Part model, mm, in its own coordinate system. Face numbers are marked on the shaded views. Round coordinates to 2 decimals unless told otherwise and drop trailing zeros. Loops run counter-clockwise (first coordinate to the right, second up) from the corner with the lowest first, then second, coordinate; pieces in that order, holes last. Notation, with made-up numbers: (-25.75, 37) -> (14.25, 37) arc R21 cw to (14.25, 54) -> close; hole circle Ø1 at (67, 75). An arc over 180 degrees is marked (long way). Use a Markdown table: item, result. Add a question column.
Item 1: Two-plate mould, pull along Z, no slides. Class the marked faces 1 and 2: pulls with the +Z half, pulls with the -Z half, needs draft (parallel to the pull), parting line crosses it, or undercut.
Item 2: Cut at C-C, the plane y = 241. List the corners of the cut face in (x, z), plus the area to 3 significant figures.
Item 3: Cut at B-B, the plane y = 73.5. List the corners of the cut face in (x, z).
Item 4: Probe line 1 (Z direction, x = 0, y = 123.5); line 2 (Z direction, x = 1.5, y = 89); line 3 (X direction, y = 176.5, z = -2). List the from-to ranges inside material, lowest first. Write a range as [from, to].
Item 5: Flat gauge pins, fed straight in: pin 1 (1.5 mm diameter, centred on x = 0, y = 121, fed in from +Z); pin 2 (12 mm diameter, centred on y = 212.5, z = -5.5, fed in from -X); pin 3 (8.5 mm diameter, centred on x = 4.5, z = 5.5, fed in from -Y); pin 4 (9 mm diameter, centred on x = 0, y = 209, fed in from -Z). Where does each tip first touch, or does it go through?
Item 6: Cut at A-A, the plane z = 0. List the corners of the cut face in (x, y).
```python
from build123d import *

# Parameters (mm, degrees)
CROQUIS2_R                 = 15
SALIENTE_EXTRUIR2_DEPTH    = 55
CORTAR_EXTRUIR1_DEPTH      = 27.5
CROQUIS6_R                 = 14
CORTAR_EXTRUIR3_DEPTH      = 54
CROQUIS7_R                 = 13.5
SALIENTE_EXTRUIR4_DEPTH    = 223
CORTAR_EXTRUIR5_REACH      = 280.808
CORTAR_EXTRUIR5_END_RADIUS = 13.5
CROQUIS9_R                 = 3.5
CORTAR_EXTRUIR6_DEPTH      = 23
CORTAR_EXTRUIR7_DEPTH      = 23
CROQUIS11_R                = 13
CORTAR_EXTRUIR8_DEPTH      = 291
REDONDEO1_R                = 10


with BuildPart() as part:
    # Croquis2 → Saliente-Extruir2 (new body)
    with BuildSketch(Plane(origin=(0, 0, 0), x_dir=(1, 0, 0), z_dir=(0, 1, 0))):
        with Locations(Location((0, 0, 0), (0, 0, 270))):
            Circle(CROQUIS2_R)
    extrude(amount=SALIENTE_EXTRUIR2_DEPTH)

    # Croquis3 → Cortar-Extruir1 (cut, symmetric)
    with BuildSketch(Plane.XY):
        with BuildLine():
            Line((-2.74026183, 0), (1.25973817, 0))
            Line((1.25973817, 0), (1.25973817, 27.763932023))
            ThreePointArc((1.25973817, 27.763932023), (-0.74026183, 33), (-2.74026183, 27.763932023))
            Line((-2.74026183, 27.763932023), (-2.74026183, 0))
        make_face()
    extrude(amount=CORTAR_EXTRUIR1_DEPTH, both=True, mode=Mode.SUBTRACT)

    # Croquis6 → Cortar-Extruir3 (cut)
    with BuildSketch(Plane(origin=(0, 0, 0), x_dir=(1, 0, 0), z_dir=(0, 1, 0))):
        with Locations(Location((0, 0, 0), (0, 0, 84.83746883))):
            Circle(CROQUIS6_R)
    extrude(amount=CORTAR_EXTRUIR3_DEPTH, mode=Mode.SUBTRACT)

    # Croquis7 → Saliente-Extruir4 (add)
    with BuildSketch(Plane(origin=(0, 55, 0), x_dir=(1, 0, 0), z_dir=(0, 1, 0))):
        with Locations(Location((0, 0, 0), (0, 0, 90))):
            Circle(CROQUIS7_R)
    extrude(amount=SALIENTE_EXTRUIR4_DEPTH)

    # Cortar-Extruir5: up to this cylinder (the profile starts inside it)
    cortar_extruir5_end = Plane(origin=(0, 255.043672, 0), z_dir=(0, -1, 0)) * Cylinder(CORTAR_EXTRUIR5_END_RADIUS, 589.616, mode=Mode.PRIVATE)
    # Croquis8 → Cortar-Extruir5 (cut, up to the surface)
    with BuildSketch(Plane.XY, mode=Mode.PRIVATE) as cortar_extruir5_sk1:
        with BuildLine():
            Line((1.73935776, 278), (-3.26064224, 278))
            Line((-3.26064224, 278), (-3.26064224, 245.330127019))
            ThreePointArc((-3.26064224, 245.330127019), (-0.76064224, 236), (1.73935776, 245.330127019))
            Line((1.73935776, 245.330127019), (1.73935776, 278))
        make_face()
    cortar_extruir5_tool1 = extrude(cortar_extruir5_sk1.sketch, amount=-CORTAR_EXTRUIR5_REACH, mode=Mode.PRIVATE) & cortar_extruir5_end
    add(cortar_extruir5_tool1.solids().sort_by_distance((-0.760642, 255.043672, 0))[0], mode=Mode.SUBTRACT)

    # Croquis9 → Cortar-Extruir6 (cut)
    with BuildSketch(Plane.XY):
        with Locations((0, 209)):
            Circle(CROQUIS9_R)
    extrude(amount=-CORTAR_EXTRUIR6_DEPTH, mode=Mode.SUBTRACT)

    # Croquis10 → Cortar-Extruir7 (cut)
    with BuildSketch(Plane(origin=(0, 0, 0), x_dir=(-1, 0, 0), z_dir=(0, 0, -1))):
        with BuildLine():
            Line((2.26064224, 271.01908507), (2.26064224, 252.48091493))
            ThreePointArc((2.26064224, 252.48091493), (0.22284696, 248.500111609), (-1.73935776, 252.518713023))
            Line((-1.73935776, 252.518713023), (-1.73935776, 270.981286977))
            ThreePointArc((-1.73935776, 270.981286977), (-2.253530287, 272.5), (-1.73935776, 274.018713023))
            Line((-1.73935776, 274.018713023), (-1.73935776, 278))
            Line((-1.73935776, 278), (2.26064224, 278))
            Line((2.26064224, 278), (2.26064224, 273.98091493))
            ThreePointArc((2.26064224, 273.98091493), (2.746469713, 272.5), (2.26064224, 271.01908507))
        make_face()
    extrude(amount=-CORTAR_EXTRUIR7_DEPTH, mode=Mode.SUBTRACT)

    # Croquis11 → Cortar-Extruir8 (cut)
    with BuildSketch(Plane(origin=(0, 0, 0), x_dir=(1, 0, 0), z_dir=(0, 1, 0))):
        with Locations(Location((0, 0, 0), (0, 0, 82.310952423))):
            Circle(CROQUIS11_R)
    extrude(amount=CORTAR_EXTRUIR8_DEPTH, mode=Mode.SUBTRACT)

    # Redondeo1
    # the kernel refuses this fillet: 10 mm, written as the material it adds along each edge
    with BuildSketch(Plane(origin=(0, 55, 0), x_dir=(0, 0, -1), z_dir=(1, 0, 0))) as redondeo1_piece_1:
        with BuildLine():
            CenterArc((23.5, 5.267826876), REDONDEO1_R, 180, 31.788330617)
            Line((13.5, 5.267826876), (13.3, 5.267826876))
            Line((13.3, 5.267826876), (13.3, 0))
            Line((13.3, 0), (13.5, -0.2))
            ThreePointArc((13.5, -0.2), (14.25, -0.2), (14.83, -0.105356538))
            Line((14.83, -0.105356538), (15, 0))
        make_face()
    revolve(axis=Axis((0, 55, 0), (0, 1, 0)))


solid = part.part
```
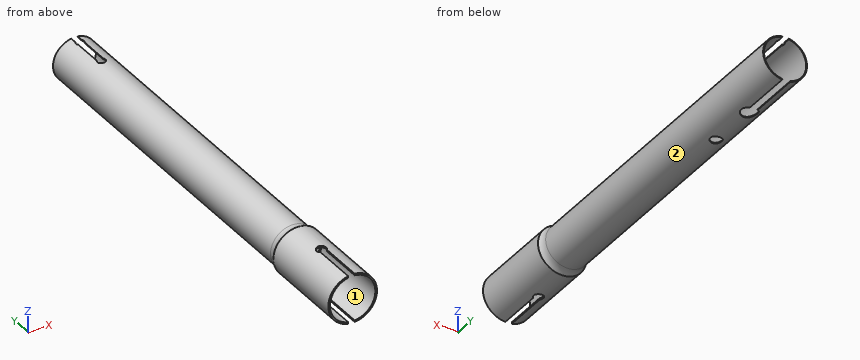
A:
| question | item | result |
|---|---|---|
| 1 | face 1 | undercut |
| 1 | face 2 | parting line crosses it |
| 2 | outline | (-5.76, -12.21) -> (-5.76, -11.65) arc R13 cw (long way) to (4.24, -12.29) -> (4.24, -12.82) arc R13.5 ccw (long way) to start |
| 2 | area | 36.5 mm^2 |
| 3 | outline | circle Ø27 at (0, 0); hole circle Ø26 at (0, 0) |
| 4 | line 1 | z = [-13.5, -13], [13, 13.5] |
| 4 | line 2 | z = [-13.42, -12.91], [12.91, 13.42] |
| 4 | line 3 | x = [-13.35, -12.85], [12.85, 13.35] |
| 5 | pin 1 | stops at z = 13.5 |
| 5 | pin 2 | stops at x = -13.5 |
| 5 | pin 3 | passes through |
| 5 | pin 4 | stops at z = -13.5 |
| 6 | outline | (-15, 0) -> (-14, 0) -> (-14, 54) -> (-13, 54) -> (-13, 278) -> (-13.5, 278) -> (-13.5, 60.27) arc R10 cw to (-15, 55) -> close; (13, 54) -> (14, 54) -> (14, 0) -> (15, 0) -> (15, 55) arc R10 cw to (13.5, 60.27) -> (13.5, 278) -> (13, 278) -> close |
